The listing builds one solid part. Answer for the finished solid, in the listing's coordinates (mm). A direction names the side the tool comes from. Round coordinates to 2 decimals unless told otherwise and drop trailing zeros. Write each loop counter-clockwise with the first axis right and the second up, starting at its lowest first coordinate (ties: lowest second). Pieces come first, ordered by that corner, then holes. Notation, with made-up numbers: M -37.75,46.25 L -13.75,46.25 A20 ccw -13.75,52.25 Z; hole C -1,-17 d9. An arc over 180 degrees is marked long. Write each question's results on one line, items separated by ' | '.
Autodesk Inventor part; units mm, degrees
ref_plane "KOLBEN_XY" through (0, 0, -387) normal (0, 0, -1) x (1, 0, 0)
ref_plane "KOLBEN_YZ" through (0, 0, -387) normal (1, 0, 0) x (0, -1, 0)
ref_plane "KOLBEN_ZX" through (0, 0, -387) normal (0, -1, 0) x (0, 0, -1)
sketch "Sketch_1" plane through (0, 0, 0) normal (1, 0, 0) x (0, 1, 0)
  line L0 (0, -387) -> (0, 0)
  line L1 (0, 0) -> (12.1, 0)
  line L2 (12.1, 0) -> (12.5, -0.4)
  line L3 (12.5, -0.4) -> (12.5, -362)
  line L4 (12.5, -362) -> (50, -362)
  line L5 (50, -362) -> (50, -387)
  line L6 (50, -387) -> (0, -387)
  line L7 (0, -387) -> (0, 0)
revolve "Revolution1" add sketch "Sketch_1" angle 360 about axis through (0, 0, -387) along (0, 0, -1)
sketch "Sketch_2" plane through (0, 0, 0) normal (1, 0, 0) x (0, 1, 0)
  line L0 (0, -1) -> (0, 32)
  line L1 (0, 32) -> (7.08, 32)
  line L2 (7.08, 32) -> (8, 31.08)
  line L3 (8, 31.08) -> (8, 5)
  line L4 (8, 5) -> (6.6425, 2.7375)
  arc A0 (6.6425, 2.7375) -> (6.5, 2.223) centre (7.5, 2.223) ccw
  line L5 (6.5, 2.223) -> (6.5, 1)
  arc A1 (6.5, 1) -> (7.5, 0) centre (7.5, 1) ccw
  line L6 (7.5, 0) -> (8, 0)
  line L7 (8, 0) -> (8, -1)
  line L8 (8, -1) -> (0, -1)
  line L9 (0, -1) -> (0, 32)
revolve "Revolution2" add sketch "Sketch_2" angle 360 about axis through (0, 0, -1) along (0, 0, -1)
thread "Thread1"
sketch "Sketch_4" plane through (0, 0, 0) normal (0, 1, 0) x (-1, 0, 0)
  line L0 (15.5, -10.4) -> (15.5, 36.6)
  line L1 (15.5, 36.6) -> (-15.5, 36.6)
  line L2 (-15.5, 36.6) -> (-15.5, -10.4)
  line L3 (-15.5, -10.4) -> (-11, -10.4)
  line L4 (-11, -10.4) -> (-11, 0)
  line L5 (-11, 0) -> (-14.5, 0)
  line L6 (-14.5, 0) -> (-14.5, 35.6)
  line L7 (-14.5, 35.6) -> (14.5, 35.6)
  line L8 (14.5, 35.6) -> (14.5, 0)
  line L9 (14.5, 0) -> (11, 0)
  line L10 (11, 0) -> (11, -10.4)
  line L11 (11, -10.4) -> (15.5, -10.4)
extrude "Extrusion1" cut sketch "Sketch_4" along normal mid plane 25
sketch "Sketch_5" plane through (0, 0, 0) normal (0, 1, 0) x (-1, 0, 0)
  line L0 (0, -10) -> (0, -10.4)
  line L1 (0, -10.4) -> (-12.5, -10.4)
  line L2 (-12.5, -10.4) -> (-12.1, -10)
  line L3 (-12.1, -10) -> (0, -10)
  line L4 (0, -10) -> (0, -10.4)
revolve "Revolution3" add sketch "Sketch_5" angle 360 about axis through (0, 0, -10) along (0, 0, 1)
ref_plane "KOLBEN_XY" through (0, 0, -387) normal (0, 0, -1) x (1, 0, 0)
ref_plane "KOLBEN_YZ" through (0, 0, -387) normal (1, 0, 0) x (0, -1, 0)
ref_plane "KOLBEN_ZX" through (0, 0, -387) normal (0, -1, 0) x (0, 0, -1)
properties part number "1808236 DFPI-100-280-ND2P-E-P(K)"
1) Section B-B (y = 0) is taken. Determine the outline of the cut face in (x, z).
Return value:
outline: M -50,-387 L 50,-387 L 50,-362 L 12.5,-362 L 12.5,-10.4 L 12.1,-10 L 11,-10 L 11,0 L 7.5,0 A1 cw 6.5,1 L 6.5,2.22 A1 cw 6.64,2.74 L 8,5 L 8,31.08 L 7.08,32 L -7.08,32 L -8,31.08 L -8,5 L -6.64,2.74 A1 cw -6.5,2.22 L -6.5,1 A1 cw -7.5,0 L -11,0 L -11,-10 L -12.1,-10 L -12.5,-10.4 L -12.5,-362 L -50,-362 Z
2) Section D-D (y = -43) is taken. Determine the outline of the cut face in (x, z).
Return value:
outline: M -25.51,-387 L 25.51,-387 L 25.51,-362 L -25.51,-362 Z
3) Find the intervals of material crossed by line 1 (Y direction, x = -1, z = -34); line 2 (Z direction, x = -45, y = 3), in increasing order.
Return value:
line 1: -12.46 to 12.46 | line 2: -387 to -362
4) Section C-C (z = -21) is taken. Determine the outline of the cut face in (x, y).
Return value:
outline: C 0,0 d25
5) A tool of negligible diameter and unlimited length cuts with its end or side. For faces 1 (the face through (3.755, 11.923, -183.731)), 2 (the face through (0.2, -12.21, -0.11)), 3 (the face through (-3.955, -5.158, 1.603)), from which of +Z, -Z, +X, -X, +Y, -Y can it reach the whole face along a straight path? Write none if from no direction.
Return value:
face 1: +Z | face 2: +Z, -Y | face 3: none
6) Each of these flat-tipped pins is pushed along its axis until it touches: pin 1 (6 mm diameter, centred on x = -9.5, z = -71, fed in from -Y); pin 2 (8.5 mm diameter, centred on y = 0.5, z = -3.5, fed in from -X); pin 3 (6 mm diameter, centred on y = -17, z = -189.5, fed in from -X); pin 4 (8.5 mm diameter, centred on y = -3, z = -5, fed in from +X). Where does it stop, or does it pass through?
Return value:
pin 1: y = -10.68 | pin 2: x = -11 | pin 3: through | pin 4: x = 11
7) Section A-A (x = 0) is taken. Determine the outline of the cut face in (y, z).
Return value:
outline: M -50,-387 L 50,-387 L 50,-362 L 12.5,-362 L 12.5,-0.4 L 12.1,0 L 7.5,0 A1 cw 6.5,1 L 6.5,2.22 A1 cw 6.64,2.74 L 8,5 L 8,31.08 L 7.08,32 L -7.08,32 L -8,31.08 L -8,5 L -6.64,2.74 A1 cw -6.5,2.22 L -6.5,1 A1 cw -7.5,0 L -12.1,0 L -12.5,-0.4 L -12.5,-362 L -50,-362 Z
8) The mould has two halves that part along Z. Classify faces 4 (the face through (-7.81, -1.73, 17.86)), 5 (the face through (-10, 10, -362)), 6 (the face through (-6.67, -0.88, 2.88)): +Z half, -Z half, draft (parallel to the pull), parting line (faces both ways), or undercut.
Return value:
face 4: draft | face 5: +Z half | face 6: undercut
